from build123d import *

# Parameters (mm, degrees)
SKETCH1_W   = 40
SKETCH1_H   = 40
SKETCH1_W_2 = 32
SKETCH1_H_2 = 32


with BuildPart() as part:
    # Sweep1: sweep along a curve in space
    with BuildLine() as sweep1_path:
        add(Edge.make_bspline(
            [(0, 0, -460), (0, 0, 500)],
            knots=[0, 0, 1, 1], degree=1))
    # Sketch1 → Sweep1 (sweep)
    with BuildSketch(Plane.XY):
        Rectangle(SKETCH1_W, SKETCH1_H)
        Rectangle(SKETCH1_W_2, SKETCH1_H_2, mode=Mode.SUBTRACT)
    sweep(path=sweep1_path.line)


solid = part.part
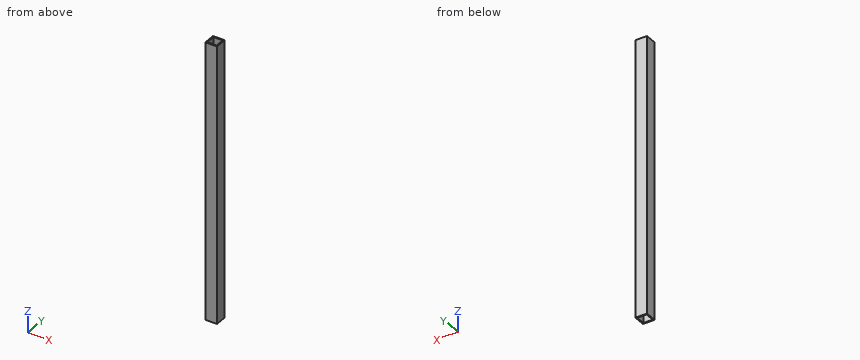
Verification items for the finished model (mm, model axes). Give positions to 0.01 mm unless a question says otherwise; leave off trailing zeros. Loops run counter-clockwise (first coordinate to the right, second up) from the corner with the lowest first, then second, coordinate; pieces in that order, holes last. Notation, with made-up numbers: (87.5, 35) - (123.5, 35) arc R20 ccw to (123.5, 70) - close; hole circle Ø11 at (-39.75, 57). An arc over 180 degrees is marked (long way). Write item = value, one per line. Start each with the question number.
Q1. Cross-section at A-A, the plane y = -4.5. Enter the section's corners in (x, z), and give its area (3 significant figures).
Q2. Cross-section at C-C, the plane z = -83.5. Enter the section's corners in (x, y), and give its area (3 significant figures).
Q3. Thickness scan on line 1 (X direction, y = -11, z = -237). Record the ranges inside material, lowest first.
Answer key:
q1.outline = (-20, -460) - (-16, -460) - (-16, 500) - (-20, 500) - close; (16, -460) - (20, -460) - (20, 500) - (16, 500) - close
q1.area = 7,680 mm^2
q2.outline = (-20, -20) - (20, -20) - (20, 20) - (-20, 20) - close; hole (-16, -16) - (16, -16) - (16, 16) - (-16, 16) - close
q2.area = 576 mm^2
q3.line_1 = -20 to -16, 16 to 20
